Autodesk Inventor part; units mm, degrees
ref_plane "YZ Plane" through (0, 0, 0) normal (1, 0, 0) x (0, 1, 0)
ref_plane "XZ Plane" through (0, 0, 0) normal (0, 1, 0) x (-1, 0, 0)
ref_plane "XY Plane" through (0, 0, 0) normal (0, 0, 1) x (1, 0, 0)
sketch "Sketch1" plane through (0, 0, 0) normal (0, 0, 1) x (1, 0, 0)
  line L0 (-27.6, 0) -> (36.8, 0)
  line L1 (0, -27.6) -> (0, 36.8)
  circle A0 centre (0, 0) radius 23
  dimension "d0" = 46
extrude "Extrusion1" add sketch "Sketch1" along normal blind 8
sketch "Sketch3" plane through (0, 0, 8) normal (0, 0, 1) x (1, 0, 0)
  circle A0 centre (0, 0) radius 23
hole "Hole1" at (0, 0, 8) direction (0, 0, -1) diameter 32 end through all
chamfer "Chamfer1" distance 5 angle 45 1 edges at (0, 16, 8)
properties part number "Bumper" material "Silicone"
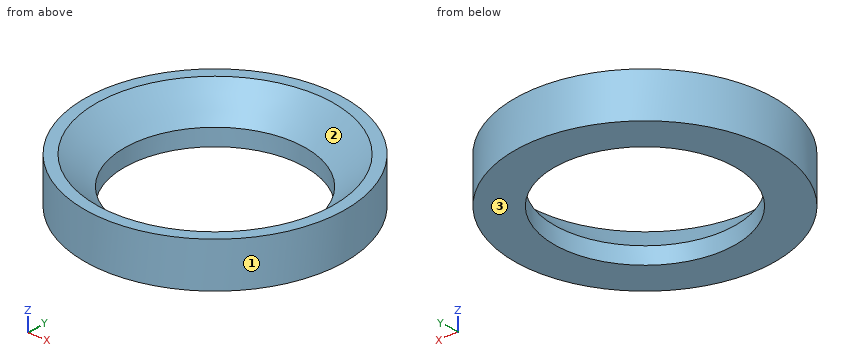
Geometry check sheet. Reference: the model listing, model coordinates, mm. Face numbers are marked on the shaded views. Round coordinates to 2 decimals unless told otherwise and drop trailing zeros. Order: outer loops, then holes, each group sorted by start corner. A loop starts at its lowest first (then second) coordinate and runs counter-clockwise, first axis right, second up. Notation, with made-up numbers: M 5,23.5 L 47,23.5 A33 ccw 47,53.5 Z; hole C 21,-28.5 d6. An arc over 180 degrees is marked long. Write item = value, one per line.
Q1. Scan lines: line 1 (X direction, y = 0, z = 0.8); line 2 (Y direction, x = -7.5, z = 2.5). Record each from-to range of solid material in increasing order.
Answer block:
line_1 = -23 to -16, 16 to 23
line_2 = -21.74 to -14.13, 14.13 to 21.74
Q2. Depth check by flat-ended pin: pin 1 Ø1.5 at (x, z) = (13, 4) entering from +Y; pin 2 Ø1.5 at (x, z) = (-7.5, 4.5) entering from -Y; pin 3 Ø2 at (x, z) = (-6.5, 5.5) entering from +Y. Enter the tip coordinate at first touch or a pass-through.
Answer block:
pin_1 = 19.47
pin_2 = -21.99
pin_3 = 22.33
Q3. Section check D-D (z = 4.75). Enter the section's corners in (x, y), plus the area to 3 significant figures.
Answer block:
outline = C 0,0 d46; hole C 0,0 d35.5
area = 672 mm^2
Q4. Section check A-A (x = 0). Enter the section's corners in (y, z).
Answer block:
outline = M -23,0 L -16,0 L -16,3 L -21,8 L -23,8 Z; M 16,0 L 23,0 L 23,8 L 21,8 L 16,3 Z
Q5. Release check for a two-part mould opening along X. For the marked faces 1, 2 and 3 record: released by +X, released by -X, zero draft, split by the parting line, or undercut.
Answer block:
face_1 = split by the parting line
face_2 = undercut
face_3 = zero draft
Q6. Section check C-C (z = 2.25). Enter the section's corners in (x, y), plus the area to 3 significant figures.
Answer block:
outline = C 0,0 d46; hole C 0,0 d32
area = 858 mm^2
